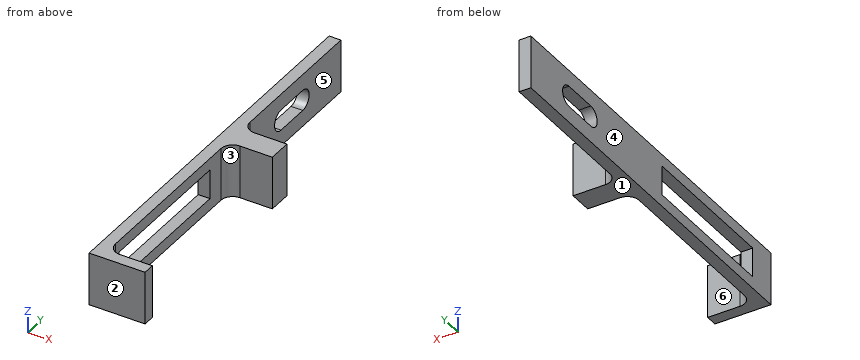
```python
from build123d import *

# Parameters (mm, degrees)
EXTRUDE_1_DEPTH     = 9
CUT_EXTRUDE_2_DEPTH = 68.284842275
SKETCH_6_W          = 5
SKETCH_6_H          = 25
CUT_EXTRUDE_3_DEPTH = 68.031708915
FILLET_1_R          = 2
SKETCH_7_W          = 7.5
SKETCH_7_H          = 4
EXTRUDE_2_DEPTH     = 9
FILLET_2_R          = 2


with BuildPart() as part:
    # Эскиз1 → Бобышка-Вытянуть1 (new body)
    with BuildSketch(Plane.XY):
        Polygon((0, 0), (9.5, 0), (9.5, 2), (2, 2), (2, 66), (0, 66), align=None)
    extrude(amount=EXTRUDE_1_DEPTH)

    # Эскиз4 → Вырез-Вытянуть2 (cut, through all)
    with BuildSketch(Plane.ZY):
        with BuildLine():
            Line((6.25, 55.52), (6.25, 49.52))
            ThreePointArc((6.25, 49.52), (4.5, 47.77), (2.75, 49.52))
            Line((2.75, 49.52), (2.75, 55.52))
            ThreePointArc((2.75, 55.52), (4.5, 57.27), (6.25, 55.52))
        make_face()
    extrude(amount=-CUT_EXTRUDE_2_DEPTH, mode=Mode.SUBTRACT)

    # Эскиз6 → Вырез-Вытянуть3 (cut, through all)
    with BuildSketch(Plane(origin=(2, 0, 0), x_dir=(0, 0, -1), z_dir=(1, 0, 0))):
        with Locations((-4.5, 17.5)):
            Rectangle(SKETCH_6_W, SKETCH_6_H)
    extrude(amount=-CUT_EXTRUDE_3_DEPTH, mode=Mode.SUBTRACT)

    # Скругление1
    fillet_1_edges = [part.edges().sort_by_distance(p)[0] for p in [
        (2, 2, 4.5),
    ]]
    fillet(fillet_1_edges, radius=FILLET_1_R)

    # Эскиз7 → Бобышка-Вытянуть2 (add)
    with BuildSketch(Plane.XY.offset(9)):
        with Locations((5.75, 37)):
            Rectangle(SKETCH_7_W, SKETCH_7_H)
    extrude(amount=-EXTRUDE_2_DEPTH)

    # Скругление2
    fillet_2_edges = [part.edges().sort_by_distance(p)[0] for p in [
        (2, 39, 4.5),
        (2, 35, 4.5),
    ]]
    fillet(fillet_2_edges, radius=FILLET_2_R)


solid = part.part
```
Source: CAD feature listing. Evaluate the final solid. Frame: model axes, mm. Face numbers are marked on the shaded views. A direction names the side the tool comes from. Give positions to 0.01 mm unless a question says otherwise; leave off trailing zeros. Loops run counter-clockwise (first coordinate to the right, second up) from the corner with the lowest first, then second, coordinate; pieces in that order, holes last. Notation, with made-up numbers: (74, 81.5) -> (89, 81.5) arc R23 ccw to (89, 108.5) -> close; hole circle Ø10 at (-4.75, 89.5). An arc over 180 degrees is marked (long way). Use a Markdown table: item, result. Add a question column.
(1) Section query A-A (y = 6.5). Output: boundary loops of the cut face in (x, z).
(2) Section query D-D (z = 8). Output: boundary loops of the cut face in (x, y).
(3) Pull-direction query (Y, two-part tool) for the marked faces 1, 2 and 3; classes: +Y half, -Y half, draft (parallel to the pull), parting line (faces both ways), or undercut.
(4) Section query B-B (x = 1.25). Output: boundary loops of the cut face in (y, z), then the cut area to 3 significant figures.
(5) Access query for the marked faces 4, 5 and 6. Directions: +Z, -Z, +X, -X, +Y, -Y. A direction counts if a zero-diameter tool reaches every point of the face in a straight line with its end or side. Return the directions, or none.
(6) First-contact query: pin 1 Ø1.6 at (x, z) = (7, 2.5) entering from +Y; pin 2 Ø4.5 at (x, z) = (5.5, 6.5) entering from +Y. Flat tips, straight axial feed; report the tip coordinate or a pass-through.
(7) Section query C-C (z = 4.5). Output: boundary loops of the cut face in (x, y).
(8) Ray query, line 1 (Y direction, x = 1, z = 4.5); line 2 (Y direction, x = 5.25, z = 7); line 3 (Z direction, x = 0.75, y = 13.5). Return the intervals inside material, ascending.
Checked values:
| question | item | result |
|---|---|---|
| 1 | outline | (0, 0) -> (2, 0) -> (2, 2) -> (0, 2) -> close; (0, 7) -> (2, 7) -> (2, 9) -> (0, 9) -> close |
| 2 | outline | (0, 0) -> (9.5, 0) -> (9.5, 2) -> (4, 2) arc R2 cw to (2, 4) -> (2, 33) arc R2 cw to (4, 35) -> (9.5, 35) -> (9.5, 39) -> (4, 39) arc R2 cw to (2, 41) -> (2, 66) -> (0, 66) -> close |
| 3 | face 1 | draft |
| 3 | face 2 | -Y half |
| 3 | face 3 | undercut |
| 4 | outline | (0, 0) -> (66, 0) -> (66, 9) -> (0, 9) -> close; hole (5, 2) -> (30, 2) -> (30, 7) -> (5, 7) -> close; hole (49.52, 2.75) -> (55.52, 2.75) arc R1.75 ccw to (55.52, 6.25) -> (49.52, 6.25) arc R1.75 ccw to start |
| 4 | area | 438 mm^2 |
| 5 | face 4 | +Z, -Z, -X, +Y, -Y |
| 5 | face 5 | +Z, -Z, +X, +Y |
| 5 | face 6 | +Z, -Z, +X |
| 6 | pin 1 | y = 39 |
| 6 | pin 2 | y = 39.15 |
| 7 | outline | (0, 0) -> (9.5, 0) -> (9.5, 2) -> (4, 2) arc R2 cw to (2, 4) -> (2, 5) -> (0, 5) -> close; (0, 30) -> (2, 30) -> (2, 33) arc R2 cw to (4, 35) -> (9.5, 35) -> (9.5, 39) -> (4, 39) arc R2 cw to (2, 41) -> (2, 47.77) -> (0, 47.77) -> close; (0, 57.27) -> (2, 57.27) -> (2, 66) -> (0, 66) -> close |
| 8 | line 1 | 0 to 5, 30 to 47.77, 57.27 to 66 |
| 8 | line 2 | 0 to 2, 35 to 39 |
| 8 | line 3 | 0 to 2, 7 to 9 |
